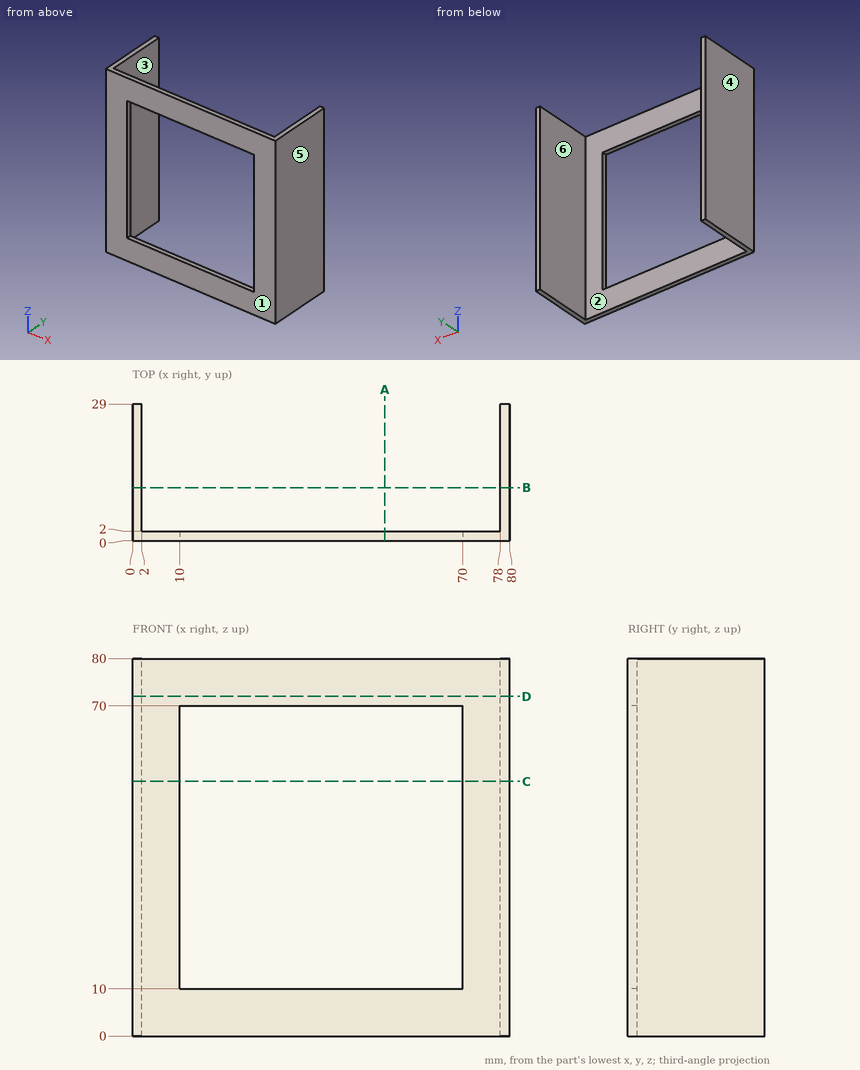
The figure shows three views and two pictorial views of one solid part (mm, origin at its lowest corner). Answer the questions. A direction names the side the tool comes from. Coordinates: 2 decimals unless noted, no trailing zeros. Loops run counter-clockwise (first coordinate to the right, second up) from the corner with the lowest first, then second, coordinate; pieces in that order, holes last. Notation, with made-up numbers: (42.5, 24.25) - (91.5, 24.25) arc R22 cw to (91.5, 31.25) - close; hole circle Ø7 at (23.25, 17). An arc over 180 degrees is marked (long way). Answer in a Markdown table with one row per item.
Q1. Straight lines are drawn through the part: line 1 along X through (y, z) = (24.75, 11); line 2 along Y through (x, z) = (6, 23.5). For each, find the intervals that lie inside material, in ascending order. Write a range as [from, to].
Here are the results:
| item | result |
|---|---|
| line 1 | x = [0, 2], [78, 80] |
| line 2 | y = [0, 2] |
Q2. Find section D-D on z = 72. Write down the section's boundary in (x, y), plus the area to 3 significant figures.
Here are the results:
| item | result |
|---|---|
| outline | (0, 0) - (80, 0) - (80, 29) - (78, 29) - (78, 2) - (2, 2) - (2, 29) - (0, 29) - close |
| area | 268 mm^2 |
Q3. Find section B-B on y = 11.25. Write down the section's boundary in (x, z).
Here are the results:
| item | result |
|---|---|
| outline | (0, 0) - (2, 0) - (2, 80) - (0, 80) - close; (78, 0) - (80, 0) - (80, 80) - (78, 80) - close |
Q4. Find section A-A on x = 53.5. Write down the section's boundary in (y, z).
Here are the results:
| item | result |
|---|---|
| outline | (0, 0) - (2, 0) - (2, 10) - (0, 10) - close; (0, 70) - (2, 70) - (2, 80) - (0, 80) - close |
Q5. The mould has two halves that part along X. Classify the marked faces 1, 2, 3 and 4: pulls with the +X half, pulls with the -X half, needs draft (parallel to the pull), parting line crosses it, or undercut.
Here are the results:
| item | result |
|---|---|
| face 1 | needs draft |
| face 2 | undercut |
| face 3 | undercut |
| face 4 | pulls with the -X half |
Q6. Find section C-C on z = 54. Write down the section's boundary in (x, y).
Here are the results:
| item | result |
|---|---|
| outline | (0, 0) - (10, 0) - (10, 2) - (2, 2) - (2, 29) - (0, 29) - close; (70, 0) - (80, 0) - (80, 29) - (78, 29) - (78, 2) - (70, 2) - close |
Q7. For the marked faces 5 and 6, determine the directions among +Z, -Z, +X, -X, +Y, -Y from which every point of the face is accessible in a straight line to the end or side of a thin tool.
Here are the results:
| item | result |
|---|---|
| face 5 | +Z, -Z, +X, +Y, -Y |
| face 6 | +Z, -Z, +Y |
Q8. Given P1, Ø1.5, axis at x = 41, z = 68, coming from the +Y side; P2, Ø10, axis at x = 12, z = 21, coming from the +Y side, each flat-ended and moving along its own axis, determine where each tip first touches the part or whether it passes through.
Here are the results:
| item | result |
|---|---|
| P1 | passes through |
| P2 | stops at y = 2 |
